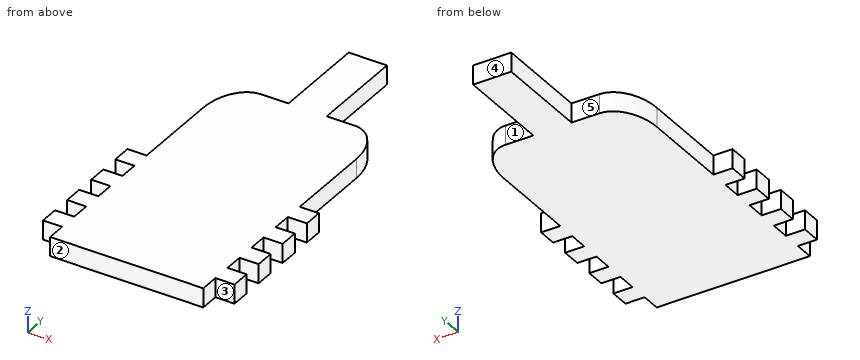
```python
from build123d import *

# Parameters (mm, degrees)
BOSS_EXTRU_1_DEPTH = 5


with BuildPart() as part:
    # Esquisse1 → Boss.-Extru.1 (new body)
    with BuildSketch(Plane.XY):
        with BuildLine():
            Line((-88.421426264, 20.834954052), (-88.421426264, 25.834954052))
            Line((-88.421426264, 25.834954052), (-93.421426264, 25.834954052))
            Line((-93.421426264, 25.834954052), (-93.421426264, 30.834954052))
            Line((-93.421426264, 30.834954052), (-88.421426264, 30.834954052))
            Line((-88.421426264, 30.834954052), (-88.421426264, 35.834954052))
            Line((-88.421426264, 35.834954052), (-93.421426264, 35.834954052))
            Line((-93.421426264, 35.834954052), (-93.421426264, 40.834954052))
            Line((-93.421426264, 40.834954052), (-88.421426264, 40.834954052))
            Line((-88.421426264, 40.834954052), (-88.421426264, 45.834954052))
            Line((-88.421426264, 45.834954052), (-93.421426264, 45.834954052))
            Line((-93.421426264, 45.834954052), (-93.421426264, 50.834954052))
            Line((-93.421426264, 50.834954052), (-88.421426264, 50.834954052))
            Line((-88.421426264, 50.834954052), (-88.421426264, 55.834954052))
            Line((-88.421426264, 55.834954052), (-93.421426264, 55.834954052))
            Line((-93.421426264, 55.834954052), (-93.421426264, 60.834954052))
            Line((-93.421426264, 60.834954052), (-88.421426264, 60.834954052))
            Line((-88.421426264, 60.834954052), (-88.421426264, 84.288786066))
            add(Edge.make_bspline(
                [(-80.671426264, 95.834954052), (-88.421426264, 95.834954052), (-88.421426264, 84.288786066)],
                knots=[3.141592654, 3.141592654, 3.141592654, 4.71238898, 4.71238898, 4.71238898], degree=2, weights=[1, 0.707106781, 1]))
            Line((-80.671426264, 95.834954052), (-73.421426264, 95.834954052))
            Line((-73.421426264, 95.834954052), (-73.421426264, 120.834954052))
            Line((-73.421426264, 120.834954052), (-63.421426264, 120.834954052))
            Line((-63.421426264, 120.834954052), (-63.421426264, 95.834954052))
            Line((-63.421426264, 95.834954052), (-56.171426264, 95.834954052))
            add(Edge.make_bspline(
                [(-48.421426264, 84.288786066), (-48.421426264, 95.834954052), (-56.171426264, 95.834954052)],
                knots=[1.570796327, 1.570796327, 1.570796327, 3.141592654, 3.141592654, 3.141592654], degree=2, weights=[1, 0.707106781, 1]))
            Line((-48.421426264, 84.288786066), (-48.421426264, 60.834954052))
            Line((-48.421426264, 60.834954052), (-43.421426264, 60.834954052))
            Line((-43.421426264, 60.834954052), (-43.421426264, 55.834954052))
            Line((-43.421426264, 55.834954052), (-48.421426264, 55.834954052))
            Line((-48.421426264, 55.834954052), (-48.421426264, 50.834954052))
            Line((-48.421426264, 50.834954052), (-43.421426264, 50.834954052))
            Line((-43.421426264, 50.834954052), (-43.421426264, 45.834954052))
            Line((-43.421426264, 45.834954052), (-48.421426264, 45.834954052))
            Line((-48.421426264, 45.834954052), (-48.421426264, 40.834954052))
            Line((-48.421426264, 40.834954052), (-43.421426264, 40.834954052))
            Line((-43.421426264, 40.834954052), (-43.421426264, 35.834954052))
            Line((-43.421426264, 35.834954052), (-48.421426264, 35.834954052))
            Line((-48.421426264, 35.834954052), (-48.421426264, 30.834954052))
            Line((-48.421426264, 30.834954052), (-43.421426264, 30.834954052))
            Line((-43.421426264, 30.834954052), (-43.421426264, 25.834954052))
            Line((-43.421426264, 25.834954052), (-48.421426264, 25.834954052))
            Line((-48.421426264, 25.834954052), (-48.421426264, 20.834954052))
            Line((-48.421426264, 20.834954052), (-88.421426264, 20.834954052))
        make_face()
    extrude(amount=BOSS_EXTRU_1_DEPTH)


solid = part.part
```
The listing builds one solid part. Answer for the finished solid, in the listing's coordinates (mm). Face numbers are marked on the shaded views. A direction names the side the tool comes from. Give positions to 0.01 mm unless a question says otherwise; leave off trailing zeros. Write each loop counter-clockwise with the first axis right and the second up, starting at its lowest first coordinate (ties: lowest second). Pieces come first, ordered by that corner, then holes. Notation, with made-up numbers: (15, -10.75) - (67, -10.75) arc R18 ccw to (67, 9.25) - close; hole circle Ø4 at (46.25, 34.5). An arc over 180 degrees is marked (long way). Use one line per item in the form item = value. Start each with the question number.
1) A tool of negligible diameter and unlimited length cuts with its end or side. For the marked faces 1, 2, 3, 4 and 5, from which of +Z, -Z, +X, -X, +Y, -Y can it reach the whole face along a straight path? Write none if from no direction.
2) Find section B-B on y = 63.5. Determine the outline of the cut face in (x, z), plus the area to 3 significant figures.
3) Consider line 1 along Y through (x, z) = (-89, 1.1); line 2 along Y through (x, z) = (-80.5, 0.45); line 3 along X through (y, z) = (32, 3.75). Determine where each line is inside the solid, lowest interval first. Write a range as from..to.
4) Find section A-A on x = -47. Determine the outline of the cut face in (y, z), plus the area to 3 significant figures.
5) Flat-ended cylindrical pins translate along their axes: pin 1 Ø2.5 at (y, z) = (32.5, 3.5) entering from -X; pin 2 Ø3 at (x, z) = (-76.5, 3.5) entering from +Y; pin 3 Ø2.5 at (y, z) = (43.5, 2.5) entering from +X. Find the tip coordinate at first contact, or state that the pin passes through.
6) Find section C-C on x = -59.5. Determine the outline of the cut face in (y, z), plus the area to 3 significant figures.
Geometry results:
q1.face_1 = +Z, -Z, +X, +Y
q1.face_2 = +Z, -Z, +X, -X, -Y
q1.face_3 = +Z, -Z, +X, -Y
q1.face_4 = +Z, -Z, +X, -X, +Y
q1.face_5 = +Z, -Z, -X, +Y
q2.outline = (-88.42, 0) - (-48.42, 0) - (-48.42, 5) - (-88.42, 5) - close
q2.area = 200 mm2
q3.line_1 = 25.83..30.83, 35.83..40.83, 45.83..50.83, 55.83..60.83
q3.line_2 = 20.83..95.83
q3.line_3 = -88.42..-48.42
q4.outline = (25.83, 0) - (30.83, 0) - (30.83, 5) - (25.83, 5) - close; (35.83, 0) - (40.83, 0) - (40.83, 5) - (35.83, 5) - close; (45.83, 0) - (50.83, 0) - (50.83, 5) - (45.83, 5) - close; (55.83, 0) - (60.83, 0) - (60.83, 5) - (55.83, 5) - close
q4.area = 100 mm2
q5.pin_1 = -88.42
q5.pin_2 = 95.83
q5.pin_3 = -48.42
q6.outline = (20.83, 0) - (95.83, 0) - (95.83, 5) - (20.83, 5) - close
q6.area = 375 mm2
